from build123d import *

# Parameters (mm, degrees)
F1_DEPTH = 12.7
F2_T     = -2.54


with BuildPart() as f1:
    # F0 (on Top) → F1 (new body)
    with BuildSketch(Plane.XY):
        with BuildLine():
            Line((0, 15), (-20, 15))
            Line((-20, 15), (-20, -15))
            Line((-20, -15), (20, -15))
            ThreePointArc((20, -15), (9.3933982822, -10.6066017178), (5, 0))
            Line((5, 0), (0, 0))
            Line((0, 0), (0, 15))
        make_face()
        with BuildLine():
            Line((20, 15), (0, 15))
            Line((0, 15), (0, 0))
            Line((0, 0), (5, 0))
            ThreePointArc((5, 0), (9.3933982822, 10.6066017178), (20, 15))
        make_face()
        with BuildLine():
            ThreePointArc((35, 0), (30.6066017178, 10.6066017178), (20, 15))
            Line((20, 15), (20, 0))
            Line((20, 0), (20, -15))
            ThreePointArc((20, -15), (30.6066017178, -10.6066017178), (35, 0))
        make_face()
        with BuildLine():
            Line((20, 0), (20, 15))
            ThreePointArc((20, 15), (9.3933982822, 10.6066017178), (5, 0))
            Line((5, 0), (20, 0))
        make_face()
        with BuildLine():
            ThreePointArc((5, 0), (9.3933982822, -10.6066017178), (20, -15))
            Line((20, -15), (20, 0))
            Line((20, 0), (5, 0))
        make_face()
    extrude(amount=F1_DEPTH)

    # F2
    f2_openings = [f1.faces().sort_by_distance(p)[0] for p in [
        (-20, 0, 6.35),
    ]]
    offset(amount=F2_T, openings=f2_openings)


solid = f1.part
Design review of the part built by this model. Coordinates are the model's own, in mm. A direction names the side the tool comes from. Coordinates: 2 decimals unless noted, no trailing zeros. Loops run counter-clockwise (first coordinate to the right, second up) from the corner with the lowest first, then second, coordinate; pieces in that order, holes last. Notation, with made-up numbers: M -11,-24 L -2,-24 A14 cw -2,-17 Z; hole C 88,6 d4. An arc over 180 degrees is marked long. Answer as CSV lines item,"result".
Item 1: For P1, Ø2, axis at y = -9.5, z = 8.5, coming from the +X side, flat-tipped, find the tip position at first contact; note if it passes through.
Answer list:
P1,"x = 32.36"
Item 2: Add section C-C on z = 5.5. State the section outline as (x, y) points.
Answer list:
outline,"M -20,-15 L 20,-15 A15 ccw 20,15 L -20,15 L -20,12.46 L 20,12.46 A12.46 cw 20,-12.46 L -20,-12.46 Z"
Item 3: Add section A-A on x = 9. State the section outline as (y, z) points, plus the area to 3 significant figures.
Answer list:
outline,"M -15,0 L 15,0 L 15,12.7 L -15,12.7 Z; hole M -12.46,2.54 L 12.46,2.54 L 12.46,10.16 L -12.46,10.16 Z"
area,"191 mm²"
Item 4: For probe 1 along Z at (x, y) = (-5, -2); probe 2 along Y at (x, z) = (6, 3.25); probe 3 along Y at (x, z) = (26.5, 9.5), list the stretches that pass through material, from the lowest coordinate up.
Answer list:
probe 1,"0 to 2.54, 10.16 to 12.7"
probe 2,"-15 to -12.46, 12.46 to 15"
probe 3,"-13.52 to -10.63, 10.63 to 13.52"
Item 5: The part is to be moulded in two halves that separate along Z. For faces 1 (the face through (32.457, -0.274, 6.297)), 2 (the face through (7, 0, 12.7)), 3 (the face through (0, -15, 6)), say which applies: pulls with the +Z half, pulls with the -Z half, needs draft (parallel to the pull), parting line crosses it, or undercut.
Answer list:
face 1,"undercut"
face 2,"pulls with the +Z half"
face 3,"needs draft"
Item 6: Add section B-B on y = -5.25. State the section outline as (x, z) points, plus the area to 3 significant figures.
Answer list:
outline,"M -20,0 L 34.05,0 L 34.05,12.7 L -20,12.7 L -20,10.16 L 31.3,10.16 L 31.3,2.54 L -20,2.54 Z"
area,"296 mm²"
Item 7: Machinability: for faces 4 (the face through (7, 0, 0)), 5 (the face through (0, -12.46, 6)), which of the approach directions +Z, -Z, +X, -X, +Y, -Y give a long, thin tool a straight path to every point of the face, cutting with its end or side? Answer none if there is none.
Answer list:
face 4,"-Z, +X, -X, +Y, -Y"
face 5,"-X"
Item 8: Add section D-D on x = 27.5. State the section outline as (y, z) points, plus the area to 3 significant figures.
Answer list:
outline,"M -12.99,0 L 12.99,0 L 12.99,12.7 L -12.99,12.7 Z; hole M -9.95,2.54 L 9.95,2.54 L 9.95,10.16 L -9.95,10.16 Z"
area,"178 mm²"
